Source: CAD feature listing. Evaluate the final solid. Frame: model axes, mm. Face numbers are marked on the shaded views. A direction names the side the tool comes from. Coordinates: 2 decimals unless noted, no trailing zeros. Write each loop counter-clockwise with the first axis right and the second up, starting at its lowest first coordinate (ties: lowest second). Pieces come first, ordered by that corner, then holes. Notation, with made-up numbers: (87, 34.5) - (95, 34.5) arc R17 ccw to (95, 43.5) - close; hole circle Ø11 at (82.5, -26.5). An arc over 180 degrees is marked (long way). One line per item, written item: value.
from build123d import *

# Parameters (mm, degrees)
F1_DEPTH = 10
F2_R     = 3
F3_R     = 1.5
F4_DEPTH = 10.001
F5_R     = 2
F6_DEPTH = 8
F7_R     = 3
F8_R     = 2
F9_DEPTH = 4.001
F10_R    = 3
F11_R    = 0.5


with BuildPart() as f1:
    # F0 (on Top) → F1 (new body)
    with BuildSketch(Plane.XY):
        Polygon((14, 12.5), (4, 12.5), (-4, 12.5), (-4, -2.5), (-14, -2.5), (-14, -12.5), (-4, -12.5), (4, -12.5), (4, 8.5), (14, 8.5), align=None)
    extrude(amount=F1_DEPTH)

    # F2
    f2_edges = [f1.edges().sort_by_distance(p)[0] for p in [
        (-4, 12.5, 5),
        (4, -12.5, 5),
    ]]
    fillet(f2_edges, radius=F2_R)

    # F3 (on face) → F4 (cut, through all)
    with BuildSketch(Plane(origin=(0, 0, 0), x_dir=(1, 0, 0), z_dir=(0, 0, -1))):
        with Locations((-9, 7.5)):
            Circle(F3_R)
    extrude(amount=-F4_DEPTH, mode=Mode.SUBTRACT)

    # F5 (on face) → F6 (cut)
    with BuildSketch(Plane(origin=(0, 0, 0), x_dir=(1, 0, 0), z_dir=(0, 0, -1))):
        with Locations((-9, 7.5)):
            Circle(F5_R)
    extrude(amount=-F6_DEPTH, mode=Mode.SUBTRACT)

    # F7
    f7_edges = [f1.edges().sort_by_distance(p)[0] for p in [
        (-14, -2.5, 5),
        (-14, -12.5, 5),
    ]]
    fillet(f7_edges, radius=F7_R)

    # F8 (on face) → F9 (cut, through all)
    with BuildSketch(Plane.XZ.offset(-8.5)):
        with Locations((9, 5)):
            Circle(F8_R)
    extrude(amount=-F9_DEPTH, mode=Mode.SUBTRACT)

    # F10
    f10_edges = [f1.edges().sort_by_distance(p)[0] for p in [
        (14, 10.5, 0),
        (14, 10.5, 10),
    ]]
    fillet(f10_edges, radius=F10_R)

    # F11
    f11_edges = [f1.edges().sort_by_distance(p)[0] for p in [
        (4, 8.5, 5),
        (-4, -2.5, 5),
    ]]
    fillet(f11_edges, radius=F11_R)


solid = f1.part
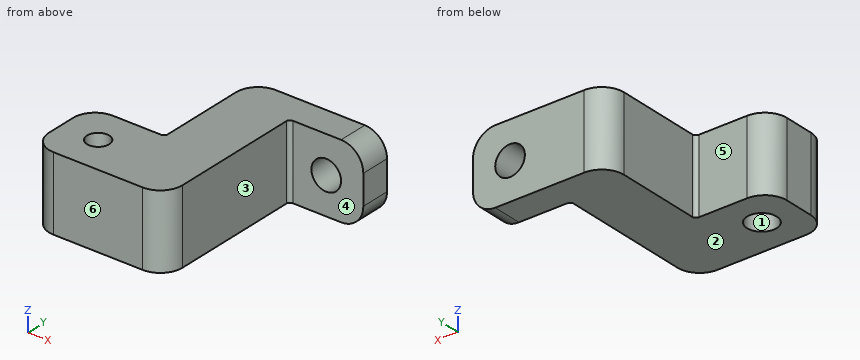
1) Section query C-C on y = -7.5. Output: boundary loops of the cut face in (x, z).
Values found:
outline: (-14, 0) - (-11, 0) - (-11, 8) - (-10.5, 8) - (-10.5, 10) - (-14, 10) - close; (-7.5, 8) - (-7, 8) - (-7, 0) - (4, 0) - (4, 10) - (-7.5, 10) - close
2) Material intervals for line 1 (Z direction, x = 9, y = 10.9); line 2 (Y direction, x = -9, z = 5.25); line 3 (Y direction, x = -9, z = 9), sorted ascending.
Values found:
line 1: 0 to 3, 7 to 10
line 2: -12.5 to -9.5, -5.5 to -2.5
line 3: -12.5 to -9, -6 to -2.5
3) Draft query along X for the marked faces 1, 2 and 3. Return one class per face: released by +X, released by -X, zero draft, split by the parting line, or undercut.
Values found:
face 1: undercut
face 2: zero draft
face 3: released by +X
4) Contact query for flat-ended pins moving along their axis: P1, Ø3.5, axis at x = -9, y = -7.5, coming from the +Z side; P2, Ø5, axis at x = 7, z = 4.5, coming from the -Y side; P3, Ø3, axis at x = -7, z = 6.5, coming from the +Y side; P4, Ø1.5, axis at y = 6, z = 1, coming from the +X side. Output: stop coordinate, or through.
Values found:
P1: z = 10
P2: y = 8.5
P3: y = -2.5
P4: x = 4
5) Section query D-D on y = 11.25. Output: boundary loops of the cut face in (x, z), then the cut area to 3 significant figures.
Values found:
outline: (-3.44, 0) - (11, 0) arc R3 ccw to (14, 3) - (14, 7) arc R3 ccw to (11, 10) - (-3.44, 10) - close; hole circle Ø4 at (9, 5)
area: 158 mm2
6) Section query A-A on z = 5. Output: boundary loops of the cut face in (x, y), then the cut area to 3 significant figures.
Values found:
outline: (-14, -9.5) arc R3 ccw to (-11, -12.5) - (1, -12.5) arc R3 ccw to (4, -9.5) - (4, 8) arc R0.5 cw to (4.5, 8.5) - (7, 8.5) - (7, 12.5) - (-1, 12.5) arc R3 ccw to (-4, 9.5) - (-4, -2) arc R0.5 cw to (-4.5, -2.5) - (-11, -2.5) arc R3 ccw to (-14, -5.5) - close; (11, 8.5) - (14, 8.5) - (14, 12.5) - (11, 12.5) - close; hole circle Ø4 at (-9, -7.5)
area: 304 mm2
7) Section query B-B on x = 9. Output: boundary loops of the cut face in (y, z).
Values found:
outline: (8.5, 0) - (12.5, 0) - (12.5, 3) - (8.5, 3) - close; (8.5, 7) - (12.5, 7) - (12.5, 10) - (8.5, 10) - close
8) Reachability of the marked faces 4, 5 and 6 from +Z, -Z, +X, -X, +Y, -Y: full face, straight path, thin tool, end or side. Return the list, or none.
Values found:
face 4: +Z, -Z, +X, -Y
face 5: +Z, -Z, -X, +Y
face 6: +Z, -Z, +X, -X, -Y
